from build123d import *

# Parameters (mm, degrees)
SKETCH1_W           = 45
SKETCH1_H           = 25
BOSS_EXTRUDE1_DEPTH = 4
SKETCH5_W           = 40.5
SKETCH5_H           = 17
CUT_EXTRUDE2_DEPTH  = 27.048032555
SKETCH6_W           = 45
SKETCH6_H           = 4.025345596
CUT_EXTRUDE3_DEPTH  = 27.048032555
SKETCH13_W          = 2.25
SKETCH13_H          = 20.974654404
BOSS_EXTRUDE3_DEPTH = 8
SKETCH16_W          = 2.25
SKETCH16_H          = 20.974654404
BOSS_EXTRUDE4_DEPTH = 8
SKETCH19_W          = 17
SKETCH19_H          = 4
BOSS_EXTRUDE5_DEPTH = 4
SKETCH21_W          = 2.25
SKETCH21_H          = 16.974654404
CUT_EXTRUDE7_DEPTH  = 27.953663944
CUT_EXTRUDE9_DEPTH  = 47.874833333
CUT_EXTRUDE14_DEPTH = 32.019125187


with BuildPart() as part:
    # Sketch1 → Boss-Extrude1 (new body)
    with BuildSketch(Plane(origin=(0, 0, 0), x_dir=(1, 0, 0), z_dir=(0, 1, 0))):
        Rectangle(SKETCH1_W, SKETCH1_H)
    extrude(amount=BOSS_EXTRUDE1_DEPTH)

    # Sketch5 → Cut-Extrude2 (cut, through all)
    with BuildSketch(Plane(origin=(0, 4, 0), x_dir=(1, 0, 0), z_dir=(0, 1, 0))):
        Rectangle(SKETCH5_W, SKETCH5_H)
    extrude(amount=-CUT_EXTRUDE2_DEPTH, mode=Mode.SUBTRACT)

    # Sketch6 → Cut-Extrude3 (cut, through all)
    with BuildSketch(Plane(origin=(0, 4, 0), x_dir=(1, 0, 0), z_dir=(0, 1, 0))):
        with Locations((0, 10.487327202)):
            Rectangle(SKETCH6_W, SKETCH6_H)
    extrude(amount=-CUT_EXTRUDE3_DEPTH, mode=Mode.SUBTRACT)

    # Sketch13 → Boss-Extrude3 (add)
    with BuildSketch(Plane(origin=(0, 4, 0), x_dir=(1, 0, 0), z_dir=(0, 1, 0))):
        with Locations((21.375, -2.012672798)):
            Rectangle(SKETCH13_W, SKETCH13_H)
    extrude(amount=-BOSS_EXTRUDE3_DEPTH)

    # Sketch16 → Boss-Extrude4 (add)
    with BuildSketch(Plane(origin=(0, 4, 0), x_dir=(1, 0, 0), z_dir=(0, 1, 0))):
        with Locations((-21.375, -2.012672798)):
            Rectangle(SKETCH16_W, SKETCH16_H)
    extrude(amount=-BOSS_EXTRUDE4_DEPTH)

    # Sketch19 → Boss-Extrude5 (add)
    with BuildSketch(Plane.XZ):
        with Locations((11.75, 10.5)):
            Rectangle(SKETCH19_W, SKETCH19_H)
    extrude(amount=BOSS_EXTRUDE5_DEPTH)

    # Sketch21 → Cut-Extrude7 (cut, through all)
    with BuildSketch(Plane(origin=(0, 4, 0), x_dir=(1, 0, 0), z_dir=(0, 1, 0))):
        with Locations((21.375, -0.012672798)):
            Rectangle(SKETCH21_W, SKETCH21_H)
    extrude(amount=-CUT_EXTRUDE7_DEPTH, mode=Mode.SUBTRACT)

    # Sketch25 → Cut-Extrude9 (cut, through all)
    with BuildSketch(Plane.ZY.offset(22.5)):
        with BuildLine():
            Line((3.314549123, -2.5), (-2.685450877, -2.5))
            ThreePointArc((-2.685450877, -2.5), (-5.185450877, 0), (-2.685450877, 2.5))
            Line((-2.685450877, 2.5), (3.314549123, 2.5))
            ThreePointArc((3.314549123, 2.5), (5.814549123, 0), (3.314549123, -2.5))
        make_face()
    extrude(amount=-CUT_EXTRUDE9_DEPTH, mode=Mode.SUBTRACT)

    # Sketch29 → Cut-Extrude14 (cut, through all)
    with BuildSketch(Plane.XY.offset(12.5)):
        with BuildLine():
            Line((6.774762471, 2), (10.174762471, 2))
            ThreePointArc((10.174762471, 2), (12.174762471, 0), (10.174762471, -2))
            Line((10.174762471, -2), (6.774762471, -2))
            ThreePointArc((6.774762471, -2), (4.774762471, 0), (6.774762471, 2))
        make_face()
    extrude(amount=-CUT_EXTRUDE14_DEPTH, mode=Mode.SUBTRACT)


solid = part.part
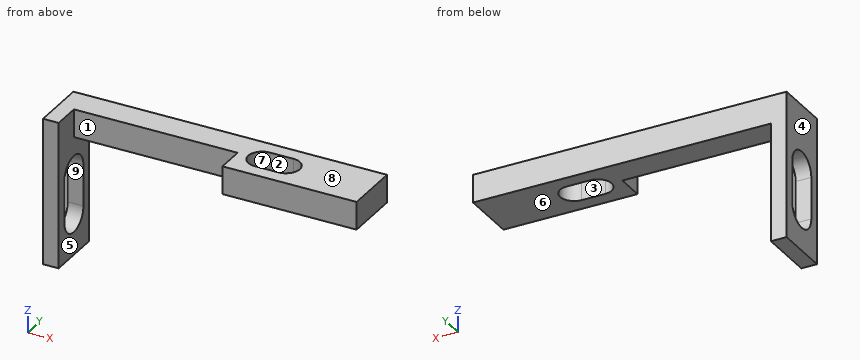
Input: part model. Units: mm. Frame: model coordinates. Face numbers are marked on the shaded views. A direction names the side the tool comes from. Coordinates: 2 decimals unless noted, no trailing zeros. Loops run counter-clockwise (first coordinate to the right, second up) from the corner with the lowest first, then second, coordinate; pieces in that order, holes last. Notation, with made-up numbers: (18.25, 27.5) - (43.25, 27.5) arc R30 ccw to (43.25, 55.5) - close; hole circle Ø10 at (27, 7). An arc over 180 degrees is marked (long way). Answer in a Markdown table with one row per item. Add a question column.
Item 1: Section query B-B on x = 9.5. Return the cut outline in (y, z), then the cut area to 3 significant figures.
Item 2: Section query A-A on z = 9.5. Return the cut outline in (x, y), then the cut area to 3 significant figures.
Item 3: Mould query, pull axis Y, two halves, no side actions, for the marked faces 1, 2, 3 and 4. Classes: released by +Y, released by -Y, zero draft, split by the parting line, or undercut.
Item 4: Access query for the marked faces 5, 6, 7, 8 and 9. Directions: +Z, -Z, +X, -X, +Y, -Y. A direction counts if a zero-diameter tool reaches every point of the face in a straight line with its end or side. Return the directions, or none.
Item 5: Contact query for flat-ended pins moving along their axis: P1, Ø3, axis at x = -8.5, z = 10, coming from the -Y side; P2, Ø12, axis at x = -13, z = -2.5, coming from the -Y side; P3, Ø2.5, axis at y = 1.5, z = -2, coming from the +X side; P4, Ø1.5, axis at x = 17.5, y = -1.5, coming from the -Z side. Output: stop coordinate, or through.
Item 6: Line query: line 1 along Z through (x, y) = (3, 3.75); line 2 along X through (y, z) = (-0.5, 10.5); line 3 along X through (y, z) = (3.5, 0.75). Output: solid intervals per line, ascending. Write a range as [from, to].
Item 7: Section query D-D on z = 5. Return the cut outline in (x, y).
Item 8: Section query C-C on y = -1.5. Return the cut outline in (x, z).
Recorded:
| question | item | result |
|---|---|---|
| 1 | outline | (-4, 8.5) - (-2, 8.5) - (-2, 12.5) - (-4, 12.5) - close; (2, 8.5) - (4, 8.5) - (4, 12.5) - (2, 12.5) - close |
| 1 | area | 16.0 mm^2 |
| 2 | outline | (-22.5, -4) - (-20.25, -4) - (-20.25, 0) - (3.25, 0) - (3.25, -4) - (22.5, -4) - (22.5, 4) - (-22.5, 4) - close; hole (6.77, -2) - (10.17, -2) arc R2 ccw to (10.17, 2) - (6.77, 2) arc R2 ccw to start |
| 2 | area | 240 mm^2 |
| 3 | face 1 | released by -Y |
| 3 | face 2 | undercut |
| 3 | face 3 | undercut |
| 3 | face 4 | zero draft |
| 4 | face 5 | -Z, -Y |
| 4 | face 6 | -Z, +X, +Y, -Y |
| 4 | face 7 | +Z, -Z |
| 4 | face 8 | +Z, +X, -X, +Y, -Y |
| 4 | face 9 | +X, -X |
| 5 | P1 | y = 0 |
| 5 | P2 | through |
| 5 | P3 | x = -20.25 |
| 5 | P4 | z = 8.5 |
| 6 | line 1 | [8.5, 12.5] |
| 6 | line 2 | [-22.5, -20.25], [3.25, 4.84], [12.11, 22.5] |
| 6 | line 3 | [-22.5, -20.25] |
| 7 | outline | (-22.5, -4) - (-20.25, -4) - (-20.25, -1.85) - (-22.5, -1.85) - close; (-22.5, 1.85) - (-20.25, 1.85) - (-20.25, 4) - (-22.5, 4) - close |
| 8 | outline | (-22.5, -8.47) - (-20.25, -8.47) - (-20.25, -4.69) - (-22.5, -4.69) - close; (-22.5, 5.31) - (-20.25, 5.31) - (-20.25, 12.5) - (-22.5, 12.5) - close; (3.25, 8.5) - (5.45, 8.5) - (5.45, 12.5) - (3.25, 12.5) - close; (11.5, 8.5) - (22.5, 8.5) - (22.5, 12.5) - (11.5, 12.5) - close |
